```python
from build123d import *

# Parameters (mm, degrees)
F0_R     = 67.471855
F1_DEPTH = 12.7
F3_DEPTH = 12.7


with BuildPart() as f1:
    # F0 (on Front) → F1 (new body)
    with BuildSketch(Plane.XZ):
        Circle(F0_R)
    extrude(amount=F1_DEPTH)

    # F2 (on face) → F3 (cut)
    with BuildSketch(Plane.XZ.offset(12.7)):
        Polygon((-12.2623, 47.785219), (-12.55971, 41.400526), (-12.55971, -47.292732), (11.735013, -47.292732), (11.735013, 47.785219), align=None)
    extrude(amount=-F3_DEPTH, mode=Mode.SUBTRACT)


solid = f1.part
```
Could you check a few things on this model? Use its own coordinates, in mm. A direction names the side the tool comes from. Coordinates: 2 decimals unless noted, no trailing zeros. Order: outer loops, then holes, each group sorted by start corner. A loop starts at its lowest first (then second) coordinate and runs counter-clockwise, first axis right, second up. Notation, with made-up numbers: M -34,42.5 L 7,42.5 A11 cw 7,58.5 Z; hole C 12.5,40 d4. An arc over 180 degrees is marked long. Use a Markdown table: item, result. Add a question column.
Q1. If I drill on L1, parallel to X at y = -4, z = -9.5; L2, parallel to X at y = -2.5, z = -24; L3, parallel to Z at x = 9, y = -6.75, over which ranges is the centre line in solid material (lowest first)?
Q2. We'd pull the mould along Z, two halves only. Please class faces 3 (the cylindrical face through (64.356, -6.261, 20.267)), 4 (the flat face through (-1, -6, -47.293)), 5 (the flat face through (14, -12.7, 1)): pulls with the +Z half, pulls with the -Z half, needs draft (parallel to the pull), parting line crosses it, or undercut.
Q3. I want a section at C-C on y = -2.5. List the corners of the cut face in (x, z) for me.
Q4. Which directions (+Z, -Z, +X, -X, +Y, -Y) give clear straight access to the entire face, cutting with the end or side of a thin tool? Please do faces 1 (the flat face through (-12.41, -6.44, 44.64)), 2 (the flat face through (14, 0, 1)).
Q5. I'm going to push flat-ended pins straight in: pin 1 (1.5 mm diameter, centred on y = -3, z = 23.5, fed in from +X); pin 2 (4 mm diameter, centred on y = -5.5, z = -7, fed in from -X); pin 3 (2 mm diameter, centred on y = -4, z = 42.5, fed in from -X). Where does each tip first touch, or does it pass through?
Q6. I want a section at A-A on z = 0. List the corners of the cut face in (x, y) for me, then the cut area to 3 significant figures.
Q7. I want a section at B-B on x = 0. List the corners of the cut face in (y, z) for me, then the cut area to 3 significant figures.
Q8. I want a section at D-D on x = -58.5. List the corners of the cut face in (y, z) for me, then the cut area to 3 significant figures.
Checked values:
| question | item | result |
|---|---|---|
| 1 | L1 | -66.8 to -12.56, 11.74 to 66.8 |
| 1 | L2 | -63.06 to -12.56, 11.74 to 63.06 |
| 1 | L3 | -66.87 to -47.29, 47.79 to 66.87 |
| 2 | face 3 | parting line crosses it |
| 2 | face 4 | undercut |
| 2 | face 5 | needs draft |
| 3 | outline | C 0,0 d134.94; hole M -12.56,-47.29 L 11.74,-47.29 L 11.74,47.79 L -12.26,47.79 L -12.56,41.4 Z |
| 4 | face 1 | +Y, -Y |
| 4 | face 2 | +Z, -Z, +X, -X, +Y |
| 5 | pin 1 | x = 63.52 |
| 5 | pin 2 | x = -67.29 |
| 5 | pin 3 | x = -53.2 |
| 6 | outline | M -67.47,-12.7 L -12.56,-12.7 L -12.56,0 L -67.47,0 Z; M 11.74,-12.7 L 67.47,-12.7 L 67.47,0 L 11.74,0 Z |
| 6 | area | 1,410 mm² |
| 7 | outline | M -12.7,-67.47 L 0,-67.47 L 0,-47.29 L -12.7,-47.29 Z; M -12.7,47.79 L 0,47.79 L 0,67.47 L -12.7,67.47 Z |
| 7 | area | 506 mm² |
| 8 | outline | M -12.7,-33.62 L 0,-33.62 L 0,33.62 L -12.7,33.62 Z |
| 8 | area | 854 mm² |
